Verification items for the finished model (mm, model axes). A direction names the side the tool comes from. Round coordinates to 2 decimals unless told otherwise and drop trailing zeros. Write each loop counter-clockwise with the first axis right and the second up, starting at its lowest first coordinate (ties: lowest second). Pieces come first, ordered by that corner, then holes. Notation, with made-up numbers: (-9, 72.5) - (10, 72.5) arc R27 cw to (10, 94.5) - close; hole circle Ø2 at (57.5, 25.25). An arc over 180 degrees is marked (long way). Answer as a JSON object with one key per item and string values.
```python
from build123d import *

# Parameters (mm, degrees)
SKETCH1_W           = 85
SKETCH1_H           = 85
BOSS_EXTRUDE1_DEPTH = 3
SKETCH2_W           = 59
SKETCH2_H           = 59
CUT_EXTRUDE1_DEPTH  = 4
DIAMETERHOLE1_D     = 7
FILLET1_R           = 3


with BuildPart() as part:
    # Sketch1 → Boss-Extrude1 (new body)
    with BuildSketch(Plane(origin=(0, 0, 0), x_dir=(0, 0, -1), z_dir=(1, 0, 0))):
        with Locations((42.5, 42.5)):
            Rectangle(SKETCH1_W, SKETCH1_H)
    extrude(amount=BOSS_EXTRUDE1_DEPTH)

    # Sketch2 → Cut-Extrude1 (cut, through all)
    with BuildSketch(Plane(origin=(0, 0, 0), x_dir=(0, 0, -1), z_dir=(1, 0, 0))):
        with Locations((55.5, 55.5)):
            Rectangle(SKETCH2_W, SKETCH2_H)
    extrude(amount=CUT_EXTRUDE1_DEPTH, mode=Mode.SUBTRACT)

    # DiameterHole1 (through all)
    with Locations(Plane(origin=(3, 0, 0), x_dir=(0, 0, -1), z_dir=(1, 0, 0))):
        with Locations((13, 74), (13, 44), (74, 13), (44, 13)):
            Hole(DIAMETERHOLE1_D / 2)

    # Fillet1
    fillet1_edges = [part.edges().sort_by_distance(p)[0] for p in [
        (1.5, 85, -26),
        (1.5, 26, -85),
        (1.5, 0, -85),
        (1.5, 0, 0),
        (1.5, 85, 0),
    ]]
    fillet(fillet1_edges, radius=FILLET1_R)


solid = part.part
```
1. Access from +Z, -Z, +X, -X, +Y, -Y to the whole of each face (thin tool, end or side, straight path). Record for faces 5 (the face through (1, 54, -26)), 6 (the face through (1.52, 0.9, -0.86)).
Completed:
{"face 5": "-Z, +X, -X, +Y", "face 6": "+Z, +X, -X, -Y"}
2. Cross-section at C-C (x = 1.4). Record the boundary of the cut face in (y, z), plus the area to 3 significant figures.
Completed:
{"outline": "(0, -82) arc R3 ccw to (3, -85) - (23, -85) arc R3 ccw to (26, -82) - (26, -26) - (82, -26) arc R3 ccw to (85, -23) - (85, -3) arc R3 ccw to (82, 0) - (3, 0) arc R3 ccw to (0, -3) - close; hole circle Ø7 at (13, -74); hole circle Ø7 at (13, -44); hole circle Ø7 at (44, -13); hole circle Ø7 at (74, -13)", "area": "3,580 mm^2"}
3. Material ranges on probe 1 along Y at (x, z) = (2.15, -13); probe 2 along Y at (x, z) = (1.4, -14); probe 3 along Z at (x, y) = (1.9, 64), recorded low to high. Write a range as from..to.
Completed:
{"probe 1": "y = 0..40.5, 47.5..70.5, 77.5..85", "probe 2": "y = 0..40.65, 47.35..70.65, 77.35..85", "probe 3": "z = -26..0"}
4. Cross-section at A-A (z = -74). Record the boundary of the cut face in (x, y), plus the area to 3 significant figures.
Completed:
{"outline": "(0, 0) - (3, 0) - (3, 9.5) - (0, 9.5) - close; (0, 16.5) - (3, 16.5) - (3, 26) - (0, 26) - close", "area": "57.0 mm^2"}
5. Cross-section at D-D (z = -13). Record the boundary of the cut face in (x, y), plus the area to 3 significant figures.
Completed:
{"outline": "(0, 0) - (3, 0) - (3, 40.5) - (0, 40.5) - close; (0, 47.5) - (3, 47.5) - (3, 70.5) - (0, 70.5) - close; (0, 77.5) - (3, 77.5) - (3, 85) - (0, 85) - close", "area": "213 mm^2"}
6. Mould release check, pull along Y, two halves, no side actions. Record for faces 1 (the face through (1, 85, -13)), 2 (the face through (1, 0, -42)), 3 (the face through (1.479, 70.583, -13.759)), 4 (the face through (1.479, 11.659, -70.767)): released by +Y, released by -Y, zero draft, split by the parting line, or undercut.
Completed:
{"face 1": "released by +Y", "face 2": "released by -Y", "face 3": "undercut", "face 4": "undercut"}
7. Go/stop test with flat-tipped pins: pin 1 (1.5 mm diameter, centred on x = 1.5, y = 45, fed in from -Z); pin 2 (1 mm diameter, centred on x = 1, z = -42, fed in from +Y). Record where each tip stops, or that it passes through.
Completed:
{"pin 1": "stops at z = -26", "pin 2": "stops at y = 26"}
8. Cross-section at B-B (y = 74). Record the boundary of the cut face in (x, z), plus the area to 3 significant figures.
Completed:
{"outline": "(0, -26) - (3, -26) - (3, -16.5) - (0, -16.5) - close; (0, -9.5) - (3, -9.5) - (3, 0) - (0, 0) - close", "area": "57.0 mm^2"}
